Read the model definition and answer for the solid it produces. Units are mm, in the model's axes. A direction names the side the tool comes from. Coordinates: 2 decimals unless noted, no trailing zeros. Loops run counter-clockwise (first coordinate to the right, second up) from the corner with the lowest first, then second, coordinate; pieces in that order, holes last. Notation, with made-up numbers: (-20.75, 28.5) - (6.25, 28.5) arc R9 ccw to (6.25, 43.5) - close; hole circle Ø10 at (56, 14). An arc over 180 degrees is marked (long way). Use CSV: the item, a comma, the result in double quotes.
Autodesk Inventor part; units mm, degrees
ref_plane "YZ Plane" through (0, 0, 0) normal (1, 0, 0) x (0, 1, 0)
ref_plane "XZ Plane" through (0, 0, 0) normal (0, 1, 0) x (-1, 0, 0)
ref_plane "XY Plane" through (0, 0, 0) normal (0, 0, 1) x (1, 0, 0)
sketch "Sketch1" plane through (0, 0, 0) normal (0, 0, 1) x (1, 0, 0)
  line L0 (43, 5.75) -> (0, 5.75)
  line L1 (0, 5.75) -> (0, 0)
  line L2 (43, 3.75) -> (43, 5.75)
  line L3 (0, 0) -> (67.7321, 0)
  line L4 (43, 3.75) -> (50, 3.75)
  line L5 (50, 3.75) -> (50, 3.5)
  line L6 (50, 3.5) -> (66, 3.5)
  line L7 (67.7321, 0) -> (67.7321, 3.5)
  line L8 (67.7321, 3.5) -> (66, 4.5)
  line L9 (66, 4.5) -> (66, 3.5)
  line L10 (66, 3.5) -> (67.7321, 3.5) construction
  dimension "d5" = 43
  dimension "d6" = 3.5
  dimension "d7" = 3.75
  dimension "d8" = 7
  dimension "d9" = 120
  dimension "d10" = 1
  dimension "d11" = 66
  dimension "d12" = 5.75
revolve "Revolution1" add sketch "Sketch1" angle 180 about axis through (0, 0, 0) along (1, 0, 0)
sketch "Sketch2" plane through (43, 5.75, 0) normal (0, 0, -1) x (-1, 0, 0)
  line L0 (-23, -1.25) -> (-23, -2.25)
  line L1 (-24.7321, -2.25) -> (-23, -1.25)
  line L2 (-24.7321, -2.25) -> (-24.7321, -9.25)
  line L3 (-24.7321, -9.25) -> (-23, -10.25)
  line L4 (-23, -10.25) -> (-23, -9.25)
  line L5 (-23, -2.25) -> (-15, -2.25)
  line L6 (-15, -2.25) -> (-15, -9.25)
  line L7 (-15, -9.25) -> (-23, -9.25)
  dimension "d14" = 8
extrude "Extrusion1" cut sketch "Sketch2" against normal blind 1.25
chamfer "Chamfer1" distance 1.25 angle 45 1 edges at (58, 0, 1.25)
sketch "Sketch3" plane through (43, 5.75, 1.25) normal (0, 0, -1) x (-1, 0, 0)
  line L0 (-23, -1.4271) -> (-23, -2.4808)
  spline S0 degree 2 poles (-24.7321, -2.4808) (-23.9862, -2.0198) (-23, -1.4271) knots 0 0 0 1 1 1 weights 1 1.008789 1
  spline S1 degree 2 poles (-23, -10.0729) (-23.9862, -9.4802) (-24.7321, -9.0192) knots 0 0 0 1 1 1 weights 1 1.008789 1
  line L1 (-23, -9.0192) -> (-23, -10.0729)
  line L2 (-23, -2.4808) -> (-24.7321, -2.4808)
  line L3 (-24.7321, -9.0192) -> (-23, -9.0192)
  point P0 (43, -5.75)
extrude "Extrusion2" cut sketch "Sketch3" against normal blind 2
mirror "Mirror1" about plane through (0, 5.75, 0) normal (-1, 0, 0)
properties part number "SpoolHandle-axis1"
Q1. For a pull along X with two mould halves and no side action, classify faces 4 (the face through (64, 0, 1.25)), 5 (the face through (-46.55, -0.08, 3.75)), 6 (the face through (66, 0, 4)), 7 (the face through (67.732, 0, 2)) as +X half, -X half, draft (parallel to the pull), parting line (faces both ways), or undercut.
Reported:
face 4,"draft"
face 5,"undercut"
face 6,"undercut"
face 7,"+X half"
Q2. Find the intervals of material crossed by probe 1 along X at (y, z) = (1.5, 5.25); probe 2 along Z at (x, y) = (11, 0.25); probe 3 along X at (y, z) = (1.5, 3.9), in increasing order. Write a range as [from, to].
Reported:
probe 1,"x = [-43, 43]"
probe 2,"z = [0, 5.74]"
probe 3,"x = [-66.56, -66], [-43, 43], [66, 66.56]"
Q3. The part is cut by section B-B on x = 9. Determine the outline of the cut face in (y, z).
Reported:
outline,"(-5.75, 0) - (5.75, 0) arc R5.75 ccw to start"
Q4. Given P1, Ø0.9, axis at x = -67, z = 1.5, coming from the -Y side; P2, Ø1.4, axis at x = -67, z = 2.5, coming from the +Y side; P3, Ø3.5, axis at x = 64, y = -1.5, coming from the -Z side, each flat-ended and moving along its own axis, determine where each tip first touches the part or whether it passes through.
Reported:
P1,"stops at y = -3.27"
P2,"stops at y = 3.27"
P3,"stops at z = 1.25"
Q5. A tool of negligible diameter and unlimited length cuts with its end or side. For faces 1 (the face through (-63, 0, 1.25)), 2 (the face through (-43, 0, 4)), 3 (the face through (-67.239, 0.064, 3.784)), from which of +Z, -Z, +X, -X, +Y, -Y can it reach the whole face along a straight path? Write none if from no direction.
Reported:
face 1,"-Z, -X, +Y, -Y"
face 2,"+Z"
face 3,"+Z, -X"
